```python
from build123d import *

# Parameters (mm, degrees)
F1_DEPTH  = 2.54
F4_DEPTH  = 6.35
F8_W      = 51.7626535147
F8_H      = 12.0121920481
F9_DEPTH  = 11.684
F10_W     = 3.2028928399
F10_H     = 21.3907221332
F11_DEPTH = 2.54
F12_W     = 3.4383758903
F12_H     = 21.8503316864
F13_DEPTH = 2.286
F15_DEPTH = 25.4
F17_DEPTH = 25.4


with BuildPart() as f1:
    # F0 (on Top) → F1 (new body)
    with BuildSketch(Plane.XY):
        Polygon((-7.5027812272, 27.2412225604), (-35.9747856855, 27.2412225604), (-35.9747856855, 13.5823562741), (-20.5845143646, 13.5823562741), align=None)
    extrude(amount=F1_DEPTH)


with BuildPart() as f2_1:
    # F2: instance of F1
    add(f1.part.mirror(Plane.XZ))


with BuildPart() as f4:
    # F3 (on Top) → F4 (new body)
    with BuildSketch(Plane.XY):
        Polygon((-27.2736139596, 6.3365907408), (-7.5153368525, 27.4984613061), (-79.1166648269, 27.4984613061), (-79.1166648269, -27.2664036602), (-7.5153368525, -27.2664036602), (-27.2736139596, -5.7910899632), align=None)
    extrude(amount=-F4_DEPTH)


with BuildPart() as f6_1:
    # F6: copy of F1
    add(f1.part.moved(Location((0, 0, -8.89))))


with BuildPart() as f7_1:
    # F7: copy of F2_1
    add(f2_1.part.moved(Location((0, 0, -8.89))))


with BuildPart() as f1_1:
    add(f1.part)

    add(f2_1.part)  # F9 merges F2_1

    add(f4.part)  # F9 merges F4

    add(f6_1.part)  # F9 merges F6_1

    add(f7_1.part)  # F9 merges F7_1
    # F8 (on offset) → F9 (join)
    with BuildSketch(Plane.XY.offset(2.794)):
        with Locations((-53.2025257125, 0.2657445148)):
            Rectangle(F8_W, F8_H)
    extrude(amount=-F9_DEPTH)

    # F10 (on Top) → F11 (cut)
    with BuildSketch(Plane.XY):
        with Locations((-77.6618160307, 16.9474571012)):
            Rectangle(F10_W, F10_H)
    extrude(amount=-F11_DEPTH, mode=Mode.SUBTRACT)

    # F12 (on Top) → F13 (cut)
    with BuildSketch(Plane.XY):
        with Locations((-77.9631473124, -16.6356083937)):
            Rectangle(F12_W, F12_H)
    extrude(amount=-F13_DEPTH, mode=Mode.SUBTRACT)

    # F14 (on offset) → F15 (cut)
    with BuildSketch(Plane.XY.offset(2.794)):
        with BuildLine():
            Line((-42.855940921, 17.7954155952), (-42.855940921, 9.5185028021))
            ThreePointArc((-42.855940921, 9.5185028021), (-39.9091769658, 10.729969596), (-38.6873239795, 13.6724421754))
            ThreePointArc((-38.6873239795, 13.6724421754), (-40.0888769364, 16.7836563698), (-43.3477644342, 17.7954155952))
            Line((-43.3477644342, 17.7954155952), (-42.855940921, 17.7954155952))
        make_face()
        with BuildLine():
            Line((-62.5399425626, 9.5185028021), (-42.855940921, 9.5185028021))
            ThreePointArc((-42.855940921, 9.5185028021), (-46.9879402117, 13.4260434851), (-43.3477644342, 17.7954155952))
            Line((-43.3477644342, 17.7954155952), (-62.5399425626, 17.7954155952))
            Line((-62.5399425626, 17.7954155952), (-62.5399425626, 17.7007548757))
            ThreePointArc((-62.5399425626, 17.7007548757), (-59.6805472176, 16.5163545436), (-58.4961468855, 13.6569591987))
            ThreePointArc((-58.4961468855, 13.6569591987), (-59.6805472176, 10.7975638537), (-62.5399425626, 9.6131635216))
            Line((-62.5399425626, 9.6131635216), (-62.5399425626, 9.5185028021))
        make_face()
        with BuildLine():
            ThreePointArc((-43.3477644342, 17.7954155952), (-46.9879402117, 13.4260434851), (-42.855940921, 9.5185028021))
            Line((-42.855940921, 9.5185028021), (-42.855940921, 17.7954155952))
            Line((-42.855940921, 17.7954155952), (-43.3477644342, 17.7954155952))
        make_face()
        with BuildLine():
            ThreePointArc((-62.5399425626, 17.7007548757), (-66.5837382396, 13.6569591987), (-62.5399425626, 9.6131635216))
            Line((-62.5399425626, 9.6131635216), (-62.5399425626, 17.7007548757))
        make_face()
        with BuildLine():
            Line((-62.5399425626, 17.7007548757), (-62.5399425626, 9.6131635216))
            ThreePointArc((-62.5399425626, 9.6131635216), (-59.6805472176, 10.7975638537), (-58.4961468855, 13.6569591987))
            ThreePointArc((-58.4961468855, 13.6569591987), (-59.6805472176, 16.5163545436), (-62.5399425626, 17.7007548757))
        make_face()
    extrude(amount=-F15_DEPTH, mode=Mode.SUBTRACT)

    # F16 (on Top) → F17 (cut)
    with BuildSketch(Plane.XY):
        with BuildLine():
            ThreePointArc((-44.1468792435, -21.0114289075), (-40.8257271545, -20.4931034722), (-39.2974471919, -17.4992643297))
            ThreePointArc((-39.2974471919, -17.4992643297), (-40.3801402653, -14.8854120279), (-42.9939925671, -13.8027189545))
            Line((-42.9939925671, -13.8027189545), (-42.9939925671, -21.0114289075))
            Line((-42.9939925671, -21.0114289075), (-44.1468792435, -21.0114289075))
        make_face()
        with BuildLine():
            Line((-42.9939925671, -21.0114289075), (-42.9939925671, -13.8027189545))
            ThreePointArc((-42.9939925671, -13.8027189545), (-46.6441517031, -16.9154955469), (-44.1468792435, -21.0114289075))
            Line((-44.1468792435, -21.0114289075), (-42.9939925671, -21.0114289075))
        make_face()
        with BuildLine():
            ThreePointArc((-44.1468792435, -21.0114289075), (-46.6441517031, -16.9154955469), (-42.9939925671, -13.8027189545))
            Line((-42.9939925671, -13.8027189545), (-62.9980564117, -13.8027189545))
            Line((-62.9980564117, -13.8027189545), (-62.9980564117, -13.8833889438))
            ThreePointArc((-62.9980564117, -13.8833889438), (-60.5064348625, -14.9154523818), (-59.4743714246, -17.407073931))
            ThreePointArc((-59.4743714246, -17.407073931), (-60.5064348625, -19.8986954802), (-62.9980564117, -20.9307589182))
            Line((-62.9980564117, -20.9307589182), (-62.9980564117, -21.0114289075))
            Line((-62.9980564117, -21.0114289075), (-44.1468792435, -21.0114289075))
        make_face()
        with BuildLine():
            ThreePointArc((-59.4743714246, -17.407073931), (-60.5064348625, -14.9154523818), (-62.9980564117, -13.8833889438))
            Line((-62.9980564117, -13.8833889438), (-62.9980564117, -20.9307589182))
            ThreePointArc((-62.9980564117, -20.9307589182), (-60.5064348625, -19.8986954802), (-59.4743714246, -17.407073931))
        make_face()
        with BuildLine():
            Line((-62.9980564117, -20.9307589182), (-62.9980564117, -13.8833889438))
            ThreePointArc((-62.9980564117, -13.8833889438), (-66.5217413989, -17.407073931), (-62.9980564117, -20.9307589182))
        make_face()
    extrude(amount=-F17_DEPTH, mode=Mode.SUBTRACT)


solid = f1_1.part
```
Could you check a few things on this model? Use its own coordinates, in mm. A direction names the side the tool comes from. Round coordinates to 2 decimals unless told otherwise and drop trailing zeros. Loops run counter-clockwise (first coordinate to the right, second up) from the corner with the lowest first, then second, coordinate; pieces in that order, holes last. Notation, with made-up numbers: (-27.75, 49.5) - (22.25, 49.5) arc R33 cw to (22.25, 87.5) - close; hole circle Ø4 at (34, 4). An arc over 180 degrees is marked (long way). Use CSV: the item, a comma, the result in double quotes.
Item 1: If we mould it in two halves opening along Y, with no side actions, what happens to faces 5 (the flat face through (-27.321, 0, -8)), 6 (the flat face through (-22, 27.241, -8)), 7 (the flat face through (-44, -27.266, -3)), 8 (the cylindrical face through (-66.52, -17.33, -3.13))? For each: pulls with the +Y half, pulls with the -Y half, needs draft (parallel to the pull), parting line crosses it, or undercut.
Here are the results:
face 5,"undercut"
face 6,"pulls with the +Y half"
face 7,"pulls with the -Y half"
face 8,"undercut"
Item 2: Will these pins go through, and if not, where does the flat tip stop? pin 1 (2 mm diameter, centred on x = -29, z = 1.5, fed in from +Y); pin 2 (0.7 mm diameter, centred on x = -8, y = -26.5, fed in from +Z); pin 3 (2 mm diameter, centred on x = -78, z = -1.5, fed in from +Y).
Here are the results:
pin 1,"stops at y = 27.24"
pin 2,"stops at z = 2.54"
pin 3,"stops at y = 6.25"
Item 3: If we section it at A-A on z = -1: List the corners of the cut face in (x, y) for me.
Here are the results:
outline,"(-79.12, -5.71) - (-76.24, -5.71) - (-76.24, -27.27) - (-7.52, -27.27) - (-27.27, -5.79) - (-27.27, 6.34) - (-7.52, 27.5) - (-76.06, 27.5) - (-76.06, 6.25) - (-79.12, 6.25) - close; hole (-63, -21.01) - (-44.15, -21.01) arc R3.7 ccw (long way) to (-42.99, -13.8) - (-63, -13.8) - (-63, -13.88) arc R3.52 ccw to (-63, -20.93) - close; hole (-62.54, 9.52) - (-42.86, 9.52) arc R4.15 ccw (long way) to (-43.35, 17.8) - (-62.54, 17.8) - (-62.54, 17.7) arc R4.04 ccw to (-62.54, 9.61) - close"
Item 4: If we section it at B-B on x = -57: List the corners of the cut face in (y, z) for me, then the cut area to 3 significant figures.
Here are the results:
outline,"(-27.27, -6.35) - (-21.01, -6.35) - (-21.01, 0) - (-27.27, 0) - close; (-13.8, -6.35) - (-5.74, -6.35) - (-5.74, -8.89) - (6.27, -8.89) - (6.27, -6.35) - (9.52, -6.35) - (9.52, 0) - (6.27, 0) - (6.27, 2.79) - (-5.74, 2.79) - (-5.74, 0) - (-13.8, 0) - close; (17.8, -6.35) - (27.5, -6.35) - (27.5, 0) - (17.8, 0) - close"
area,"313 mm²"
Item 5: For faces 1 (the flat face through (-78, 17, -2.54)), 2 (the flat face through (-28, -13.582, -8)), 3 (the flat face through (-28, 13.582, 1)), 4 (the flat face through (-25, 21, 2.54)), which set-ups out of +Z, -Z, +X, -X, +Y, -Y let a thin tool reach every point of the face, with its end or its side?
Here are the results:
face 1,"+Z, -X, +Y"
face 2,"-Z, +X, -X"
face 3,"+Z, +X, -X"
face 4,"+Z, +X, -X, +Y"
Item 6: I need wall thicknesses on L1, parallel to Y at x = -62, z = -6; L2, parallel to Y at x = -27.5, z = 2.25; L3, parallel to X at y = 4, z = -6.25. Which ranges of each line are inside material? Lowest first, please. Write a range as [from, to].
Here are the results:
L1,"y = [-27.27, -21.01], [-13.8, 9.52], [17.8, 27.5]"
L2,"y = [-27.24, -13.58], [-5.74, 6.27], [13.58, 27.24]"
L3,"x = [-79.12, -27.27]"
